For this review, take the finished solid that the model builds, in its own axes (mm). Face numbers are marked on the shaded views. Round coordinates to 2 decimals unless told otherwise and drop trailing zeros. Order: outer loops, then holes, each group sorted by start corner. A loop starts at its lowest first (then second) coordinate and runs counter-clockwise, first axis right, second up.
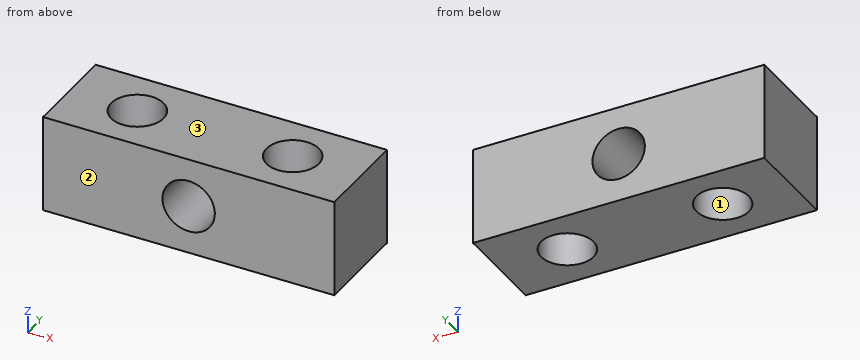
from build123d import *

# Parameters (mm, degrees)
SKETCH1_W           = 38.1
SKETCH1_H           = 12.7
BOSS_EXTRUDE1_DEPTH = 12.7
SKETCH2_R           = 3.429
CUT_EXTRUDE1_DEPTH  = 12.7
SKETCH3_R           = 3.429
CUT_EXTRUDE2_DEPTH  = 12.7


with BuildPart() as part:
    # Sketch1 → Boss-Extrude1 (new body)
    with BuildSketch(Plane.XY):
        Rectangle(SKETCH1_W, SKETCH1_H)
    extrude(amount=BOSS_EXTRUDE1_DEPTH)

    # Sketch2 → Cut-Extrude1 (cut)
    with BuildSketch(Plane.XY.offset(12.7)):
        with Locations((10.16, 0)):
            Circle(SKETCH2_R)
    cut_extrude1 = extrude(amount=-CUT_EXTRUDE1_DEPTH, mode=Mode.SUBTRACT)

    # Sketch3 → Cut-Extrude2 (cut)
    with BuildSketch(Plane(origin=(0, 6.35, 0), x_dir=(1, 0, 0), z_dir=(0, 1, 0))):
        with Locations(Location((0, -6.35, 0), (0, 0, 270))):
            Circle(SKETCH3_R)
    extrude(amount=-CUT_EXTRUDE2_DEPTH, mode=Mode.SUBTRACT)

    # Mirror1: Cut-Extrude1 across plane
    add(cut_extrude1.mirror(Plane(origin=(0, 0, 0), x_dir=(0, 0, 1), z_dir=(1, 0, 0))), mode=Mode.SUBTRACT)


solid = part.part
(1) Wall thickness on L1, parallel to X at y = 1.25, z = 6.35; L2, parallel to X at y = 2.5, z = 4.5; L3, parallel to Y at x = -10.16, z = 6.25: over which ranges is each line inside the solid? List them lowest first.
(2) Add section B-B on z = 6.35. Give the boundary of the cut face in (x, y).
(3) Draft analysis for pull direction Y (two halves, no side actions). For the marked faces 1, 2 and 3, state which applies: pulls with the +Y half, pulls with the -Y half, needs draft (parallel to the pull), parting line crosses it, or undercut.
(4) Add section A-A on y = 0. Give the boundary of the cut face in (x, z).
(5) Add section D-D on y = -4.75. Give the boundary of the cut face in (x, z), plus the area to 3 significant figures.
(6) Add section C-C on x = 0. Give the boundary of the cut face in (y, z), plus the area to 3 significant figures.
Here are the results:
1. L1: x = -19.05 to -13.35, -6.97 to -3.43, 3.43 to 6.97, 13.35 to 19.05
1. L2: x = -19.05 to -12.51, -7.81 to -2.89, 2.89 to 7.81, 12.51 to 19.05
1. L3: y = -6.35 to -3.43, 3.43 to 6.35
2. outline: (-19.05, -6.35) - (-3.43, -6.35) - (-3.43, 6.35) - (-19.05, 6.35) - close; (3.43, -6.35) - (19.05, -6.35) - (19.05, 6.35) - (3.43, 6.35) - close; hole circle Ø6.86 at (-10.16, 0); hole circle Ø6.86 at (10.16, 0)
3. face 1: undercut
3. face 2: pulls with the -Y half
3. face 3: needs draft
4. outline: (-19.05, 0) - (-13.59, 0) - (-13.59, 12.7) - (-19.05, 12.7) - close; (-6.73, 0) - (6.73, 0) - (6.73, 12.7) - (-6.73, 12.7) - close; (13.59, 0) - (19.05, 0) - (19.05, 12.7) - (13.59, 12.7) - close; hole circle Ø6.86 at (0, 6.35)
5. outline: (-19.05, 0) - (19.05, 0) - (19.05, 12.7) - (-19.05, 12.7) - close; hole circle Ø6.86 at (0, 6.35)
5. area: 447 mm2
6. outline: (-6.35, 0) - (6.35, 0) - (6.35, 2.92) - (-6.35, 2.92) - close; (-6.35, 9.78) - (6.35, 9.78) - (6.35, 12.7) - (-6.35, 12.7) - close
6. area: 74.2 mm2
